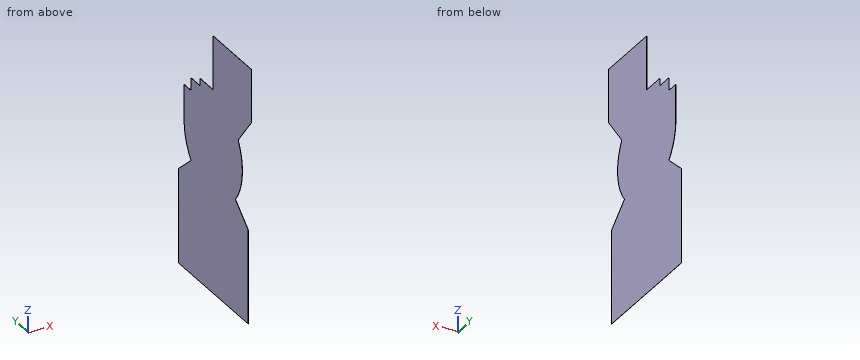
from build123d import *

# Parameters (mm, degrees)
PAD_DEPTH = 1


with BuildPart() as part:
    # Sketch → Pad (new body)
    with BuildSketch(Plane.YZ.offset(500)):
        with BuildLine():
            ThreePointArc((-427.08313, 260), (-498.445232, -39.399887), (-380.9308, -323.869921))
            Line((-380.9308, -323.869921), (-600, -507.690796))
            Line((-600, -507.690796), (-600, -1400))
            Line((-600, -1400), (600, -1400))
            Line((600, -1400), (600, -507.690796))
            Line((600, -507.690796), (380.9308, -323.869921))
            ThreePointArc((380.9308, -323.869921), (463.899857, -186.539332), (499.099189, -30))
            Line((499.099189, 340), (499.099189, -30))
            Line((380, 340), (499.099189, 340))
            Line((380, 460), (380, 340))
            Line((230, 460), (380, 460))
            Line((230, 530), (230, 460))
            Line((0, 530), (230, 530))
            Line((0, 1040), (0, 530))
            Line((-658.874021, 1040), (0, 1040))
            Line((-658.874021, 1040), (-658.874021, 540))
            Line((-427.08313, 260), (-658.874021, 540))
        make_face()
    extrude(amount=PAD_DEPTH)


solid = part.part
Verification items for the finished model (mm, model axes). Give positions to 0.01 mm unless a question says otherwise; leave off trailing zeros. Write each loop counter-clockwise with the first axis right and the second up, starting at its lowest first coordinate (ties: lowest second). Pieces come first, ordered by that corner, then holes. Notation, with made-up numbers: M -25,62 L 15,62 A15 cw 15,68 Z; hole C 26.5,-13.75 d2. An arc over 180 degrees is marked long. Put each result on its own line as item: value. Start each with the question number.
1. Section check D-D (z = -898). Record the cut outline in (x, y).
2. Section check C-C (y = -450). Record the cut outline in (x, z), and give its area (3 significant figures).
3. Section check A-A (y = 474). Record the cut outline in (x, z).
4. Section check B-B (x = 500.65). Record the cut outline in (y, z).
5. Scan lines: line 1 along Z through (x, y) = (500.55, -445); line 2 along Y through (x, z) = (500.5, -1239); line 3 along Z through (x, y) = (500.3, 265). Record each from-to range of solid material in increasing order. Write a range as [from, to].
Answer list:
1. outline: M 500,-600 L 501,-600 L 501,600 L 500,600 Z
2. outline: M 500,-1400 L 501,-1400 L 501,-381.83 L 500,-381.83 Z; M 500,-217.94 L 501,-217.94 L 501,217.94 L 500,217.94 Z; M 500,287.68 L 501,287.68 L 501,1040 L 500,1040 Z
2. area: 2,210 mm2
3. outline: M 500,-1400 L 501,-1400 L 501,-401.96 L 500,-401.96 Z; M 500,-159.14 L 501,-159.14 L 501,340 L 500,340 Z
4. outline: M -658.87,540 L -427.08,260 A500 ccw -380.93,-323.87 L -600,-507.69 L -600,-1400 L 600,-1400 L 600,-507.69 L 380.93,-323.87 A500 ccw 499.1,-30 L 499.1,340 L 380,340 L 380,460 L 230,460 L 230,530 L 0,530 L 0,1040 L -658.87,1040 Z
5. line 1: [-1400, -377.63], [-227.98, 227.98], [281.64, 1040]
5. line 2: [-600, 600]
5. line 3: [-1400, 460]
